from build123d import *

# Parameters (mm, degrees)
SKETCH_1_W          = 30
SKETCH_1_H          = 30
EXTRUDE_1_DEPTH     = 40
SKETCH_2_R          = 2.45
EXTRUDE_2_DEPTH     = 19
SKETCH_3_R          = 4.95
EXTRUDE_3_DEPTH     = 9
SKETCH_4_W          = 15.6
SKETCH_4_H          = 15.6
CUT_EXTRUDE_1_DEPTH = 1
SKETCH_5_W          = 2.75
SKETCH_5_H          = 15.6
CUT_EXTRUDE_2_DEPTH = 3
FILLET_1_R          = 3


with BuildPart() as part:
    # 草图1 → 凸台-拉伸1 (new body)
    with BuildSketch(Plane(origin=(0, 0, 0), x_dir=(1, 0, 0), z_dir=(0, 1, 0))):
        Rectangle(SKETCH_1_W, SKETCH_1_H)
    extrude(amount=EXTRUDE_1_DEPTH)

    # 草图2 → 凸台-拉伸2 (add)
    with BuildSketch(Plane.XZ):
        with Locations(Location((0, 0, 0), (0, 0, 270))):
            Circle(SKETCH_2_R)
    extrude(amount=EXTRUDE_2_DEPTH)

    # 草图3 → 凸台-拉伸3 (add)
    with BuildSketch(Plane.XZ.offset(19)):
        with Locations(Location((0, 0, 0), (0, 0, 270))):
            Circle(SKETCH_3_R)
    extrude(amount=EXTRUDE_3_DEPTH)

    # 草图4 → 切除-拉伸1 (cut)
    with BuildSketch(Plane.XY.offset(15)):
        with Locations((0, 17.8)):
            Rectangle(SKETCH_4_W, SKETCH_4_H)
    extrude(amount=-CUT_EXTRUDE_1_DEPTH, mode=Mode.SUBTRACT)

    # 草图5 → 切除-拉伸2 (cut)
    with BuildSketch(Plane.XY.offset(14)):
        with Locations((-6.425, 17.8)):
            Rectangle(SKETCH_5_W, SKETCH_5_H)
        with Locations((6.425, 17.8)):
            Rectangle(SKETCH_5_W, SKETCH_5_H)
    extrude(amount=-CUT_EXTRUDE_2_DEPTH, mode=Mode.SUBTRACT)

    # 圆角1
    fillet_1_edges = [part.edges().sort_by_distance(p)[0] for p in [
        (0, 0, 2.45),
    ]]
    fillet(fillet_1_edges, radius=FILLET_1_R)


solid = part.part
The model under review builds one solid part; all positions refer to its coordinate system, in mm. A direction names the side the tool comes from. Round coordinates to 2 decimals unless told otherwise and drop trailing zeros. Write each loop counter-clockwise with the first axis right and the second up, starting at its lowest first coordinate (ties: lowest second). Pieces come first, ordered by that corner, then holes. Notation, with made-up numbers: M -19.75,38 L 24.25,38 A20 ccw 24.25,74 Z; hole C 0.25,26.5 d7. An arc over 180 degrees is marked long. Answer as CSV lines item,"result". Start each with the question number.
Q1. The part is to be moulded in two halves that separate along Y. For faces 1 (the face through (0, 29, 15)), 2 (the face through (0, -28, 0)), 3 (the face through (-5.05, 18, 13)), say which applies: +Y half, -Y half, draft (parallel to the pull), parting line (faces both ways), or undercut.
Q2. Consider section B-B, the plane y = 17. Give the boundary of the cut face in (x, z).
Q3. Consider section C-C, the plane x = 0. Give the boundary of the cut face in (y, z), then the cut area to 3 significant figures.
Q4. Consider section A-A, the plane z = 0. Give the boundary of the cut face in (x, y).
Q5. Consider section D-D, the plane z = -12.5. Give the boundary of the cut face in (x, y), then the cut area to 3 significant figures.
Q6. Clearance check with flat-ended pins moving along their axes: P1, Ø2, axis at x = -6, y = 18, coming from the +Z side; P2, Ø3, axis at x = 3, z = 12, coming from the -Y side; P3, Ø1, axis at x = -2.5, y = -2, coming from the -Z side. State where each tip first meets the part, or that it passes through.
Q7. Wall thickness on line 1 along X through (y, z) = (15, 11.75); line 2 along Y through (x, z) = (12.75, -2.25); line 3 along Z through (x, y) = (0.75, 24): over which ranges is each line inside the solid? List them lowest first.
Q8. Tool access review of faces 4 (the face through (15, 20, 0)), 5 (the face through (5.05, 18, 13)), 6 (the face through (-7, 0, 0)), 7 (the face through (-2, -19, -2)), 8 (the face through (-15, 20, 0)): name each direction out of +Z, -Z, +X, -X, +Y, -Y from which nothing blocks a thin tool from reaching the whole face with its end or side.
Result set:
1,face 1,"draft"
1,face 2,"-Y half"
1,face 3,"undercut"
2,outline,"M -15,-15 L 15,-15 L 15,15 L 7.8,15 L 7.8,11 L 5.05,11 L 5.05,14 L -5.05,14 L -5.05,11 L -7.8,11 L -7.8,15 L -15,15 Z"
3,outline,"M -28,-4.95 L -19,-4.95 L -19,-2.45 L -3,-2.45 A3 cw 0,-5.45 L 0,-15 L 40,-15 L 40,15 L 25.6,15 L 25.6,14 L 10,14 L 10,15 L 0,15 L 0,5.45 A3 cw -3,2.45 L -19,2.45 L -19,4.95 L -28,4.95 Z"
3,area,"1,370 mm²"
4,outline,"M -15,0 L -5.45,0 A3 cw -2.45,-3 L -2.45,-19 L -4.95,-19 L -4.95,-28 L 4.95,-28 L 4.95,-19 L 2.45,-19 L 2.45,-3 A3 cw 5.45,0 L 15,0 L 15,40 L -15,40 Z"
5,outline,"M -15,0 L 15,0 L 15,40 L -15,40 Z"
5,area,"1,200 mm²"
6,P1,"stops at z = 14"
6,P2,"stops at y = 0"
6,P3,"stops at z = -1.77"
7,line 1,"x = -15 to -7.8, -5.05 to 5.05, 7.8 to 15"
7,line 2,"y = 0 to 40"
7,line 3,"z = -15 to 14"
8,face 4,"+Z, -Z, +X, +Y, -Y"
8,face 5,"+Z"
8,face 6,"-Y"
8,face 7,"none"
8,face 8,"+Z, -Z, -X, +Y, -Y"
